Autodesk Inventor part; units mm, degrees
ref_plane "YZ Plane" through (0, 0, 0) normal (1, 0, 0) x (0, 1, 0)
ref_plane "XZ Plane" through (0, 0, 0) normal (0, 1, 0) x (-1, 0, 0)
ref_plane "XY Plane" through (0, 0, 0) normal (0, 0, 1) x (1, 0, 0)
sketch "Schizzo1" plane through (0, 0, 0) normal (0, 0, 1) x (1, 0, 0)
  line L0 (-16, 25) -> (16, 25)
  line L1 (-16, 25) -> (-16, 32)
  line L2 (-16, 32) -> (-19, 32)
  line L3 (-19, 32) -> (-19, 0)
  line L4 (16, 25) -> (16, 32)
  line L5 (16, 32) -> (19, 32)
  line L6 (19, 32) -> (19, 0)
  line L7 (-19, 0) -> (19, 0)
  point P0 (0, 0)
  point P1 (0, 0)
  dimension "d2" = 7
  dimension "d3" = 3
  dimension "d4" = 3
  dimension "d5" = 7
  dimension "d6" = 50
  dimension "d7" = 32
  dimension "d8" = 38
revolve "Rivoluzione1" add sketch "Schizzo1" angle 360 about axis through (-19, 0, 0) along (1, 0, 0)
sketch "Schizzo3" plane through (-19, 0, 0) normal (-1, 0, 0) x (0, 0, 1)
  point P0 (0, 0)
sketch "Schizzo4" plane through (19, 0, 0) normal (1, 0, 0) x (0, 0, -1)
  circle A0 centre (0, 0) radius 14.75
  dimension "d13" = 29.5
extrude "Estrusione2" add sketch "Schizzo4" along normal blind 15
sketch "Schizzo5" plane through (34, 0, 0) normal (1, 0, 0) x (0, 0, -1)
  circle A0 centre (0, 0) radius 8
  dimension "d16" = 16
extrude "Estrusione3" add sketch "Schizzo5" along normal blind 25
thread "Filettatura1"
sketch "Schizzo6" plane through (-19, 0, 0) normal (-1, 0, 0) x (0, 0, 1)
  circle A0 centre (0, 0) radius 10
  dimension "d24" = 20
extrude "Estrusione4" add sketch "Schizzo6" along normal blind 40
chamfer "Smusso1" distance 0.75 angle 45 3 edges at (34, 0, 14.75) (59, 0, 8) (-59, 0, -10)
properties part number "Puleggia minore" material "Alluminio 6061"
Read the model definition and answer for the solid it produces. Units are mm, in the model's axes. A direction names the side the tool comes from. Coordinates: 2 decimals unless noted, no trailing zeros. Write each loop counter-clockwise with the first axis right and the second up, starting at its lowest first coordinate (ties: lowest second). Pieces come first, ordered by that corner, then holes. Notation, with made-up numbers: (-37.5, -29.75) - (0.5, -29.75) arc R36 cw to (0.5, 5.25) - close; hole circle Ø7 at (79, 71.25). An arc over 180 degrees is marked (long way). Answer as a JSON object with one key per item and string values. Group by question number.
1. A cutting plane is placed at D-D (z = -22). Determine the outline of the cut face in (x, y).
2. Which of the six approach directions +Z, -Z, +X, -X, +Y, -Y give full straight-line access (tool end or side, diameter ignored) to faces 4 (the cylindrical face through (45.96, 7.81, 1.73)), 5 (the flat face through (-16, -19.1, -16.4)), 6 (the cylindrical face through (-17.52, -6.94, 31.24)), 7 (the cylindrical face through (-38.35, 9.76, -2.17))?
3. A cutting plane is placed at C-C (x = -42). Determine the outline of the cut face in (y, z).
4. A cutting plane is placed at A-A (y = 28.5). Determine the outline of the cut face in (x, z), plus the area to 3 significant figures.
5. Each of these flat-tipped pins is pushed along its axis until it touches: P1, Ø19, axis at y = 11.5, z = 8, coming from the +X side; P2, Ø3, axis at x = 4, z = 3, coming from the -Y side; P3, Ø4, axis at x = 20.5, y = -9, coming from the -Z side; P4, Ø10, axis at y = 20, z = -0.5, coming from the -X side. Where does it stop, or does it pass through?
6. Consider L1, parallel to X at y = 17.5, z = 26; L2, parallel to X at y = -5.5, z = 16.5; L3, parallel to Z at x = 0.5, y = 15. Determine where each line is inside the solid, lowest interval first. Write a range as [from, to].
7. The mould has two halves that part along X. Classify faces 1 (the flat face through (16, -19.1, -16.4)), 2 (the flat face through (59, 0, 0)), 3 (the flat face through (-59, 0, 0)): +X half, -X half, draft (parallel to the pull), parting line (faces both ways), or undercut.
Worked out:
{
 "1": {"outline": "(-19, -23.24) - (-16, -23.24) - (-16, -11.87) - (16, -11.87) - (16, -23.24) - (19, -23.24) - (19, 23.24) - (16, 23.24) - (16, 11.87) - (-16, 11.87) - (-16, 23.24) - (-19, 23.24) - close"},
 "2": {"face 4": "+X", "face 5": "none", "face 6": "+X, -X", "face 7": "-X"},
 "3": {"outline": "circle Ø20 at (0, 0)"},
 "4": {"outline": "(-19, -14.55) - (-16, -14.55) - (-16, 14.55) - (-19, 14.55) - close; (16, -14.55) - (19, -14.55) - (19, 14.55) - (16, 14.55) - close", "area": "175 mm²"},
 "5": {"P1": "stops at x = 59", "P2": "stops at y = -24.95", "P3": "stops at z = -31.07", "P4": "stops at x = -19"},
 "6": {"L1": "x = [-19, -16], [16, 19]", "L2": "x = [-19, 19]", "L3": "z = [-20, 20]"},
 "7": {"face 1": "undercut", "face 2": "+X half", "face 3": "-X half"}
}
